```python
from build123d import *

# Parameters (mm, degrees)
CROQUIS1_W              = 19.5
CROQUIS1_H              = 40.6
SALIENTE_EXTRUIR2_DEPTH = 5
CROQUIS3_R              = 1.95
CORTAR_EXTRUIR1_DEPTH   = 10


with BuildPart() as part:
    # Croquis1 → Saliente-Extruir2 (new body)
    with BuildSketch(Plane.XY):
        Polygon((-14.75, 33.1), (14.75, 33.1), (14.75, 0), (14.75, -38.1), (-14.75, -38.1), (-14.75, 0), align=None)
        Rectangle(CROQUIS1_W, CROQUIS1_H, mode=Mode.SUBTRACT)
    extrude(amount=SALIENTE_EXTRUIR2_DEPTH)

    # Croquis3 → Cortar-Extruir1 (cut)
    with BuildSketch(Plane.XY.offset(5)):
        with Locations((-5.05, 24.2)):
            Circle(CROQUIS3_R)
        with Locations((4.85, 24.2)):
            Circle(CROQUIS3_R)
        with Locations((-5.05, -24.1)):
            Circle(CROQUIS3_R)
        with Locations((4.85, -24.1)):
            Circle(CROQUIS3_R)
    extrude(amount=-CORTAR_EXTRUIR1_DEPTH, mode=Mode.SUBTRACT)


solid = part.part
```
Could you check a few things on this model? Use its own coordinates, in mm. A direction names the side the tool comes from. Round coordinates to 2 decimals unless told otherwise and drop trailing zeros. Loops run counter-clockwise (first coordinate to the right, second up) from the corner with the lowest first, then second, coordinate; pieces in that order, holes last. Notation, with made-up numbers: M -9,1.25 L 49,1.25 A28 ccw 49,30.25 Z; hole C -30,-12 d11. An arc over 180 degrees is marked long. Write item = value, one per line.
1. I need wall thicknesses on probe 1 along Y at (x, z) = (4.85, 3.55); probe 2 along X at (y, z) = (2.5, 2.85); probe 3 along Y at (x, z) = (-7.75, 2.8). Which ranges of each line are inside material? Lowest first, please.
Results below:
probe_1 = -38.1 to -26.05, -22.15 to -20.3, 20.3 to 22.25, 26.15 to 33.1
probe_2 = -14.75 to -9.75, 9.75 to 14.75
probe_3 = -38.1 to -20.3, 20.3 to 33.1
2. Will this pin go through, and if not, where does the flat tip stop? P1, Ø2.5, axis at x = -5.05, y = 24.2, coming from the -Z side.
Results below:
P1 = through
3. I want a section at A-A, the plane y = 14. Write out the boundary of the cut face in (x, z), and give its area (3 significant figures).
Results below:
outline = M -14.75,0 L -9.75,0 L -9.75,5 L -14.75,5 Z; M 9.75,0 L 14.75,0 L 14.75,5 L 9.75,5 Z
area = 50.0 mm²
4. I want a section at B-B, the plane z = 1.95. Write out the boundary of the cut face in (x, y), and give its area (3 significant figures).
Results below:
outline = M -14.75,-38.1 L 14.75,-38.1 L 14.75,33.1 L -14.75,33.1 Z; hole M -9.75,-20.3 L 9.75,-20.3 L 9.75,20.3 L -9.75,20.3 Z; hole C -5.05,-24.1 d3.9; hole C -5.05,24.2 d3.9; hole C 4.85,-24.1 d3.9; hole C 4.85,24.2 d3.9
area = 1,260 mm²
5. I want a section at D-D, the plane y = -24.1. Write out the boundary of the cut face in (x, z).
Results below:
outline = M -14.75,0 L -7,0 L -7,5 L -14.75,5 Z; M -3.1,0 L 2.9,0 L 2.9,5 L -3.1,5 Z; M 6.8,0 L 14.75,0 L 14.75,5 L 6.8,5 Z
6. Thinking about a two-plate mould opening in Y: for faces 3 (the face through (-4.002, -22.456, 2.535)), 4 (the face through (4.427, 22.296, 2.535)), 5 (the face through (0, -38.1, 2)), 6 (the face through (14.75, -3, 2)), which applies, +Y half, -Y half, draft (parallel to the pull), parting line (faces both ways), or undercut?
Results below:
face_3 = undercut
face_4 = undercut
face_5 = -Y half
face_6 = draft
7. Which directions (+Z, -Z, +X, -X, +Y, -Y) give clear straight access to the entire face, cutting with the end or side of a thin tool? Please do faces 1 (the face through (9.75, 0, 2)), 2 (the face through (10, -2, 0)).
Results below:
face_1 = +Z, -Z
face_2 = -Z, +X, -X, +Y, -Y
8. I want a section at C-C, the plane x = -5.05. Write out the boundary of the cut face in (y, z).
Results below:
outline = M -38.1,0 L -26.05,0 L -26.05,5 L -38.1,5 Z; M -22.15,0 L -20.3,0 L -20.3,5 L -22.15,5 Z; M 20.3,0 L 22.25,0 L 22.25,5 L 20.3,5 Z; M 26.15,0 L 33.1,0 L 33.1,5 L 26.15,5 Z
